CAD build for the part. Positions are in the model's coordinates, mm. A direction names the side the tool comes from. Coordinates: 2 decimals unless noted, no trailing zeros. Order: outer loops, then holes, each group sorted by start corner. A loop starts at its lowest first (then second) coordinate and runs counter-clockwise, first axis right, second up. Notation, with made-up numbers: M 75.25,78 L 131.25,78 A17 ccw 131.25,82 Z; hole C 39.5,72 d6. An arc over 180 degrees is marked long. Write item = value, one per line.
from build123d import *

# Parameters (mm, degrees)
SKETCH2_W               = 1.9
SKETCH2_H               = 3.2
CUT_EXTRUDE1_DEPTH      = 6.45
CUT_EXTRUDE1_DEPTH_BACK = 6.45


with BuildPart() as part:
    # Sketch1 → Revolve1 (revolve)
    with BuildSketch(Plane.XY):
        Polygon((0, 0), (3, 1.732050808), (3, 21.432050808), (5.45, 23.882050808), (5.45, 24.732050808), (0, 24.732050808), align=None)
    revolve(axis=Axis((0, 24.732050808, 0), (0, -1, 0)))

    # Sketch2 → Cut-Extrude1 (cut, two sides)
    with BuildSketch(Plane.XY) as cut_extrude1_sk:
        with Locations((0, 24.732050808)):
            Rectangle(SKETCH2_W, SKETCH2_H)
    extrude(amount=CUT_EXTRUDE1_DEPTH, mode=Mode.SUBTRACT)
    extrude(cut_extrude1_sk.sketch, amount=-CUT_EXTRUDE1_DEPTH_BACK, mode=Mode.SUBTRACT)


solid = part.part
(1) Tool access for faces 5 (the face through (-0.95, 24, 0)), 6 (the face through (-3, 12, 0)), 7 (the face through (3, 24.732, 0)): list every direction of +Z, -Z, +X, -X, +Y, -Y with a clear straight run to the whole face (end or side of a thin tool).
Evaluation:
face_5 = +Z, -Z, +Y
face_6 = -Y
face_7 = +Z, -Z, +X, -X, +Y
(2) Wall check: line 1 (X direction, y = 23.25, z = 4); line 2 (Z direction, x = 4.5, y = 23.5); line 3 (Z direction, x = -1.75, y = 13.75). Give the ranges that are in metal, low to high. Write a range as from..to.
Evaluation:
line_1 = -2.69..-0.95, 0.95..2.69
line_2 = -2.33..2.33
line_3 = -2.44..2.44
(3) Slice it at A-A, the plane y = 9.25. Write the cut outline in (x, z).
Evaluation:
outline = C 0,0 d6
(4) Pull direction X, two halves, no side cores. Call faces 1 (the face through (-0.11, 0.3, -0.51)), 2 (the face through (0, 23.132, 0)), 3 (the face through (-3, 24.732, 0)), 4 (the face through (0.95, 24, 0)): +X half, -X half, draft (parallel to the pull), parting line (faces both ways), or undercut.
Evaluation:
face_1 = parting line
face_2 = undercut
face_3 = draft
face_4 = undercut
(5) Pin check, flat tips, straight feed: pin 1 Ø1.8 at (y, z) = (24, 1.5) entering from +X; pin 2 Ø3 at (y, z) = (19.5, 1.5) entering from -X; pin 3 Ø1.5 at (x, y) = (3, 12) entering from +Z. Stop position of each tip, or through.
Evaluation:
pin_1 = 5.42
pin_2 = -3
pin_3 = 1.98
